Autodesk Inventor part; units mm, degrees
ref_plane "Work Plane2" through (-42.9985, 19.9999, -14.0003) normal (1, 0, 0) x (0, 1, 0)
ref_plane "YZ Plane" through (0, 0, 0) normal (1, 0, 0) x (0, 1, 0)
ref_plane "XZ Plane" through (0, 0, 0) normal (0, 1, 0) x (-1, 0, 0)
ref_plane "Work Plane1" through (-73.1749, 241, 50) normal (-1, 0, 0) x (0, 0, 1)
sketch "Sketch1" plane through (-73.1749, 241, 50) normal (-1, 0, 0) x (0, 0, 1)
  line L0 (-50, -231) -> (-64, -231)
  line L1 (-50, -231) -> (-50, -20)
  arc A0 (-40, -10) -> (-50, -20) centre (-40, -20) ccw
  line L2 (0, -10) -> (-40, -10)
  line L3 (0, 0) -> (0, -10)
  line L4 (-64, 0) -> (0, 0)
  line L5 (-64, 0) -> (-64, -231)
  circle A1 centre (-21.5, -69.8271) radius 4 construction
  line L6 (-11, -56.6947) -> (-11, -84.1618) construction
  line L7 (-8, -23.5901) -> (-50, -23.5901)
  line L8 (-50, -23.5901) -> (-50, -33.5901)
  line L9 (-30, -33.5901) -> (-8, -33.5901)
  line L10 (-8, -33.5901) -> (-8, -23.5901)
  line L11 (-50, -183.5901) -> (-8, -183.5901)
  line L12 (-8, -183.5901) -> (-8, -173.5901)
  line L13 (-8, -173.5901) -> (-30, -173.5901)
  line L14 (-50, -173.5901) -> (-50, -183.5901)
  line L15 (-50, -33.5901) -> (-40, -33.5901)
  line L16 (-40, -43.5901) -> (-40, -163.5901)
  line L17 (-40, -173.5901) -> (-50, -173.5901)
  line L18 (-50, -173.5901) -> (-50, -33.5901)
  arc A2 (-30, -33.5901) -> (-40, -43.5901) centre (-30, -43.5901) ccw
  arc A3 (-40, -163.5901) -> (-30, -173.5901) centre (-30, -163.5901) ccw
  point P0 (-50, -241)
  dimension "d0" = 10
  dimension "d1" = 10
  dimension "d2" = 42
  dimension "d3" = 10
  dimension "d4" = 140
  dimension "d5" = 10
  dimension "d18" = 0
ref_plane "Work Plane2" through (-42.9985, 19.9999, -14.0003) normal (1, 0, 0) x (0, 1, 0)
extrude "Extrusion1" add sketch "Sketch1" against normal up to surface (30.1764 mm away) contours L1 L7 L10 L9 A2 L16 A3 L13 L12 L11
sketch "Sketch2" plane through (-73.1749, 57.4099, 0) normal (0, -1, 0) x (1, 0, 0)
  line L0 (30.1764, 0) -> (30.1764, 42)
  line L1 (0, 42) -> (30.1764, 42)
  line L2 (0, 0) -> (0, 42)
  line L3 (0, 0) -> (30.1764, 0)
  circle A0 centre (5, 36) radius 3
  line L4 (0, 42) -> (30.1764, 42)
  point P0 (73.1749, 0)
  dimension "d8" = 6
  dimension "d19" = 6
extrude "Extrusion2" cut sketch "Sketch2" against normal through all contours A0
sketch "Sketch3" plane through (-73.1749, 77.4099, 10) normal (0, 0, 1) x (1, 0, 0)
  arc A0 (7, 91.7198) -> (7, 90.4353) centre (5.7, 91.0776) ccw
  circle A1 centre (5, 96.0295) radius 1.4
  circle A2 centre (5, 8.0376) radius 1.4
  point P0 (73.1749, -77.4099)
hole "Hole1" at (-68.1749, 173.4393, 10) at (-68.1749, 85.4474, 10) direction (0, 0, -1) diameter 2.9 end through all both
properties part number "15_Opentrons_Additional_Slide"
Model file for the job. Use its own axes, mm. A direction names the side the tool comes from. Round coordinates to 2 decimals unless told otherwise and drop trailing zeros. Loops run counter-clockwise (first coordinate to the right, second up) from the corner with the lowest first, then second, coordinate; pieces in that order, holes last. Notation, with made-up numbers: M 58.5,84.5 L 72.5,84.5 A20 cw 72.5,122.5 Z; hole C -34,-34.75 d10. An arc over 180 degrees is marked long. Put each result on its own line as item: value. Start each with the question number.
Item 1: Cut at D-D (y = 131). List the corners of the cut face in (x, z), then the cut area to 3 significant figures.
Item 2: Cut at A-A (z = 26). List the corners of the cut face in (x, y).
Item 3: Cut at B-B (x = -59). List the corners of the cut face in (y, z).
Item 4: Drill centre lines: line 1 along Y through (x, z) = (-70, 25); line 2 along Y through (x, z) = (-67, 2.5); line 3 along Z through (x, y) = (-61, 120). Where is each one in solid material? Low to high.
Item 5: 3-axis set-ups, long thin cutter, end or side, ignore diameter. For faces 1 (the face through (-58.3, 70.42, 12.85)), 2 (the face through (-42.998, 138, 5)): which of +Z, -Z, +X, -X, +Y, -Y reach the whole face in a straight line?
Item 6: Mould opens along Z. For faces 3 (the face through (-58, 136, 0)), 4 (the face through (-58, 67.41, 31)), 5 (the face through (-70.386, 62.34, 38.028)) say: released by +Z, released by -Z, zero draft, split by the parting line, or undercut.
Item 7: Drop a flat-ended pin along its axis: P1, Ø1.5, axis at x = -68, y = 127, coming from the +Z side. Give the stop position or say it passes through.
Item 8: Cut at C-C (z = 36). List the corners of the cut face in (x, y).
Answer block:
1. outline: M -73.17,0 L -43,0 L -43,10 L -73.17,10 Z
1. area: 302 mm2
2. outline: M -73.17,57.41 L -43,57.41 L -43,67.41 L -73.17,67.41 Z; M -73.17,207.41 L -43,207.41 L -43,217.41 L -73.17,217.41 Z
3. outline: M 57.41,0 L 217.41,0 L 217.41,42 L 207.41,42 L 207.41,20 A10 cw 197.41,10 L 77.41,10 A10 cw 67.41,20 L 67.41,42 L 57.41,42 Z
4. line 1: 57.41 to 67.41, 207.41 to 217.41
4. line 2: 57.41 to 84.6, 86.3 to 172.59, 174.29 to 217.41
4. line 3: 0 to 10
5. face 1: +Z, +X, -X
5. face 2: +Z, -Z, +X, +Y, -Y
6. face 3: released by -Z
6. face 4: zero draft
6. face 5: undercut
7. P1: z = 10
8. outline: M -73.17,57.41 L -71.17,57.41 L -71.17,67.41 L -73.17,67.41 Z; M -73.17,207.41 L -71.17,207.41 L -71.17,217.41 L -73.17,217.41 Z; M -65.17,57.41 L -43,57.41 L -43,67.41 L -65.17,67.41 Z; M -65.17,207.41 L -43,207.41 L -43,217.41 L -65.17,217.41 Z
